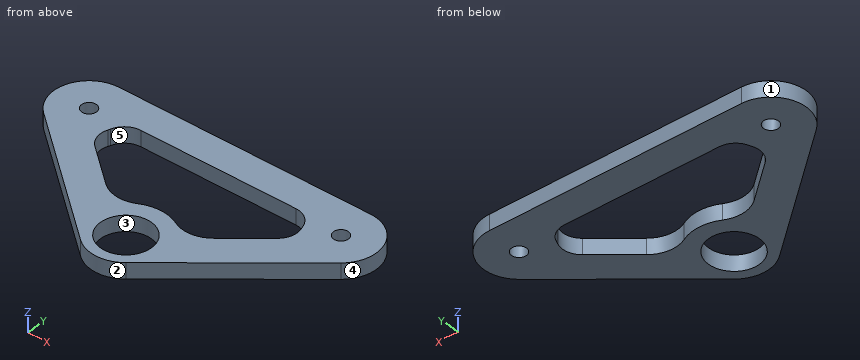
```python
from build123d import *

# Parameters (mm, degrees)
SKETCH_1_R      = 6.5
SKETCH_1_R_2    = 1.9
EXTRUDE_1_DEPTH = 4


with BuildPart() as part:
    # 草图1 → 凸台-拉伸1 (new body)
    with BuildSketch(Plane.XY):
        with BuildLine():
            Line((-32.173866611, 35.997079607), (32.173866611, 35.997079607))
            ThreePointArc((32.173866611, 35.997079607), (40.631100198, 30.075260897), (37.958955098, 20.102679619))
            Line((37.958955098, 20.102679619), (5.785088487, -6.894399988))
            ThreePointArc((5.785088487, -6.894399988), (0, -9), (-5.785088487, -6.894399988))
            Line((-5.785088487, -6.894399988), (-37.958955098, 20.102679619))
            ThreePointArc((-37.958955098, 20.102679619), (-40.631100198, 30.075260897), (-32.173866611, 35.997079607))
        make_face()
        Circle(SKETCH_1_R, mode=Mode.SUBTRACT)
        with Locations((32.173866611, 26.997079607)):
            Circle(SKETCH_1_R_2, mode=Mode.SUBTRACT)
        with Locations((-32.173866611, 26.997079607)):
            Circle(SKETCH_1_R_2, mode=Mode.SUBTRACT)
        with BuildLine():
            Line((23.341207762, 18.280191535), (13.760949221, 10.241400126))
            ThreePointArc((13.760949221, 10.241400126), (9.471070536, 8.415299285), (4.891665276, 9.290942408))
            ThreePointArc((4.891665276, 9.290942408), (0, 10.5), (-4.891665276, 9.290942408))
            ThreePointArc((-4.891665276, 9.290942408), (-9.471070536, 8.415299285), (-13.760949221, 10.241400126))
            Line((-13.760949221, 10.241400126), (-23.341207762, 18.280191535))
            ThreePointArc((-23.341207762, 18.280191535), (-24.979589386, 20.904182513), (-24.760576213, 23.989900618))
            ThreePointArc((-24.760576213, 23.989900618), (-24.656325645, 24.26091846), (-24.561979302, 24.535541145))
            ThreePointArc((-24.561979302, 24.535541145), (-22.746291761, 27.040117307), (-19.804549734, 27.997079607))
            Line((-19.804549734, 27.997079607), (19.804549734, 27.997079607))
            ThreePointArc((19.804549734, 27.997079607), (22.746291761, 27.040117307), (24.561979302, 24.535541145))
            ThreePointArc((24.561979302, 24.535541145), (24.656325645, 24.26091846), (24.760576213, 23.989900618))
            ThreePointArc((24.760576213, 23.989900618), (24.979589386, 20.904182513), (23.341207762, 18.280191535))
        make_face(mode=Mode.SUBTRACT)
    extrude(amount=EXTRUDE_1_DEPTH)


solid = part.part
```
Input: part model. Units: mm. Frame: model coordinates. Face numbers are marked on the shaded views. A direction names the side the tool comes from. Give positions to 0.01 mm unless a question says otherwise; leave off trailing zeros. Write each loop counter-clockwise with the first axis right and the second up, starting at its lowest first coordinate (ties: lowest second). Pieces come first, ordered by that corner, then holes. Notation, with made-up numbers: (76.25, -5) - (101.25, -5) arc R22 ccw to (101.25, 16) - close; hole circle Ø5 at (0, -39.75). An arc over 180 degrees is marked (long way). Write item = value, one per line. Start each with the question number.
1) Cut plane A-A (x = 0). Return loops of the section in (y, z).
2) Cut plane C-C (x = -19). Return loops of the section in (y, z).
3) Draft query along X for the marked faces 1, 2 and 3. Return one class per face: pulls with the +X half, pulls with the -X half, needs draft (parallel to the pull), parting line crosses it, or undercut.
4) Reachability of the marked faces 4 and 5 from +Z, -Z, +X, -X, +Y, -Y: full face, straight path, thin tool, end or side. Return the list, or none.
5) Cut plane D-D (z = 0.65). Return loops of the section in (x, y), and give its area (3 significant figures).
6) Material intervals for L1, parallel to Y at x = 0, z = 2.25; L2, parallel to Y at x = 1.5, z = 0.4; L3, parallel to X at y = 9, z = 1.55, sorted ascending. Write a range as [from, to].
7) Pin query (flat end, axial travel): pin 1 (2 mm diameter, centred on x = -10, z = 1.5, fed in from -Y). Return the tip coordinate at first contact, or that it passes through.
8) Cut plane B-B (y = 5). Return loops of the section in (x, z), and give its area (3 significant figures).
Answers follow:
q1.outline = (-9, 0) - (-6.5, 0) - (-6.5, 4) - (-9, 4) - close; (6.5, 0) - (10.5, 0) - (10.5, 4) - (6.5, 4) - close; (28, 0) - (36, 0) - (36, 4) - (28, 4) - close
q2.outline = (4.19, 0) - (14.64, 0) - (14.64, 4) - (4.19, 4) - close; (28, 0) - (36, 0) - (36, 4) - (28, 4) - close
q3.face_1 = pulls with the -X half
q3.face_2 = parting line crosses it
q3.face_3 = undercut
q4.face_4 = +Z, -Z, +X
q4.face_5 = +Z, -Z
q5.outline = (-37.96, 20.1) - (-5.79, -6.89) arc R9 ccw to (5.79, -6.89) - (37.96, 20.1) arc R9 ccw to (32.17, 36) - (-32.17, 36) arc R9 ccw to start; hole circle Ø3.8 at (-32.17, 27); hole (-24.76, 23.99) arc R5 ccw to (-23.34, 18.28) - (-13.76, 10.24) arc R8 ccw to (-4.89, 9.29) arc R10.5 cw to (4.89, 9.29) arc R8 ccw to (13.76, 10.24) - (23.34, 18.28) arc R5 ccw to (24.76, 23.99) arc R8 cw to (24.56, 24.54) arc R5 ccw to (19.8, 28) - (-19.8, 28) arc R5 ccw to (-24.56, 24.54) arc R8 cw to start; hole circle Ø13 at (0, 0); hole circle Ø3.8 at (32.17, 27)
q5.area = 1,510 mm^2
q6.L1 = [-9, -6.5], [6.5, 10.5], [28, 36]
q6.L2 = [-8.87, -6.32], [6.32, 10.39], [28, 36]
q6.L3 = [-24.73, -11.73], [-5.51, 5.51], [11.73, 24.73]
q7.pin_1 = -4.2
q8.outline = (-19.96, 0) - (-4.15, 0) - (-4.15, 4) - (-19.96, 4) - close; (4.15, 0) - (19.96, 0) - (19.96, 4) - (4.15, 4) - close
q8.area = 126 mm^2
